from build123d import *

# Parameters (mm, degrees)
F0_R     = 38.1
F1_DEPTH = 12.7
F2_R     = 22.225
F3_DEPTH = 12.7


with BuildPart() as f1:
    # F0 (on Front) → F1 (new body)
    with BuildSketch(Plane.XZ):
        Circle(F0_R)
        Polygon((-6.35, 0), (-6.35, 6.35), (0, 6.35), (6.35, 6.35), (6.35, -6.35), (-6.35, -6.35), align=None, mode=Mode.SUBTRACT)
    extrude(amount=F1_DEPTH)

    # F2 (on Top) → F3 (join)
    with BuildSketch(Plane.XY):
        with BuildLine():
            ThreePointArc((26.144302, 0), (26.417088, 5.50585), (28.997098, 10.377435))
            ThreePointArc((28.997098, 10.377435), (0, 73.191364), (-28.997098, 10.377435))
            ThreePointArc((-28.997098, 10.377435), (-26.417088, 5.50585), (-26.144302, 0))
            Line((-26.144302, 0), (-6.061642, 0))
            Line((-6.061642, 0), (-6.061642, -6.35))
            Line((-6.061642, -6.35), (6.417282, -6.35))
            Line((6.417282, -6.35), (6.417282, 0))
            Line((6.417282, 0), (26.144302, 0))
        make_face()
        with Locations((0, 35.091364)):
            Circle(F2_R, mode=Mode.SUBTRACT)
    extrude(amount=-F3_DEPTH)


solid = f1.part
Geometry check sheet. Reference: the model listing, model coordinates, mm. A direction names the side the tool comes from. Round coordinates to 2 decimals unless told otherwise and drop trailing zeros. Order: outer loops, then holes, each group sorted by start corner. A loop starts at its lowest first (then second) coordinate and runs counter-clockwise, first axis right, second up. Notation, with made-up numbers: M 28,47.5 L 38,47.5 A31 cw 38,73.5 Z; hole C 61.5,-1.75 d3. An arc over 180 degrees is marked long. Answer in a Markdown table with one row per item. Add a question column.
Item 1: Sectioned sample at A-A, the plane x = 0. Enter the section's corners in (y, z), plus the area to 3 significant figures.
Item 2: Sectioned sample at B-B, the plane y = 56. Enter the section's corners in (x, z).
Item 3: Material ranges on L1, parallel to Y at x = 8.5, z = 35.5; L2, parallel to Z at x = 29, y = -0.5, recorded low to high. Write a range as [from, to].
Item 4: Sectioned sample at D-D, the plane z = -32.5. Enter the section's corners in (x, y).
Item 5: Draft check along X on faces 4 (the face through (0, -9, -6.35)), 5 (the face through (26.397, 5.431, -6.261)), 6 (the face through (8, -12.7, 1)), 7 (the face through (1.214, 73.172, -6.261)). Enter one of: released by +X, released by -X, zero draft, split by the parting line, or undercut.
Item 6: Set-up check for faces 1 (the face through (-0.5, 12.7, -12.7)), 2 (the face through (0, -6, 6.35)), 3 (the face through (0, -6.35, -3)): record each of +Z, -Z, +X, -X, +Y, -Y from which the full face is reachable in a straight line by a thin tool's end or side.
Item 7: Sectioned sample at C-C, the plane x = -33. Enter the section's corners in (y, z), plus the area to 3 significant figures.
Item 8: Depth check by flat-ended pin: pin 1 Ø4 at (y, z) = (-5.5, 2.5) entering from +X; pin 2 Ø5 at (x, z) = (3, -1.5) entering from -Y; pin 3 Ø10 at (y, z) = (15, -5) entering from -X; pin 4 Ø4 at (y, z) = (-9, -0.5) entering from -X. Enter the tip coordinate at first touch or a pass-through.
Filled in:
| question | item | result |
|---|---|---|
| 1 | outline | M -12.7,-38.1 L 0,-38.1 L 0,-12.7 L 12.87,-12.7 L 12.87,0 L -6.35,0 L -6.35,-6.35 L -12.7,-6.35 Z; M -12.7,6.35 L 0,6.35 L 0,38.1 L -12.7,38.1 Z; M 57.32,-12.7 L 73.19,-12.7 L 73.19,0 L 57.32,0 Z |
| 1 | area | 1,210 mm² |
| 2 | outline | M -31.85,-12.7 L -7.54,-12.7 L -7.54,0 L -31.85,0 Z; M 7.54,-12.7 L 31.85,-12.7 L 31.85,0 L 7.54,0 Z |
| 3 | L1 | y = [-12.7, 0] |
| 3 | L2 | z = [-24.71, 24.71] |
| 4 | outline | M -19.88,-12.7 L 19.88,-12.7 L 19.88,0 L -19.88,0 Z |
| 5 | face 4 | undercut |
| 5 | face 5 | released by +X |
| 5 | face 6 | zero draft |
| 5 | face 7 | split by the parting line |
| 6 | face 1 | -Z, +X, -X, +Y |
| 6 | face 2 | +Y, -Y |
| 6 | face 3 | -Y |
| 7 | outline | M -12.7,-19.04 L 0,-19.04 L 0,19.04 L -12.7,19.04 Z; M 16.05,-12.7 L 54.13,-12.7 L 54.13,0 L 16.05,0 Z |
| 7 | area | 967 mm² |
| 8 | pin 1 | stops at x = 38.1 |
| 8 | pin 2 | stops at y = -6.35 |
| 8 | pin 3 | stops at x = -34.98 |
| 8 | pin 4 | stops at x = -38.1 |
